```python
from build123d import *

# Parameters (mm, degrees)
EXTRUDE_1_DEPTH          = 11.5
CUT_EXTRUDE_1_DEPTH      = 220.099292559
CUT_EXTRUDE_1_DEPTH_BACK = 220.099292559
CUT_EXTRUDE_3_DEPTH      = 10


with BuildPart() as part:
    # 草图2 → 凸台-拉伸1 (new body)
    with BuildSketch(Plane(origin=(0, 0, 0), x_dir=(1, 0, 0), z_dir=(0, 1, 0))):
        with BuildLine():
            Line((-167, 104), (167, 104))
            ThreePointArc((167, 104), (185.03122292, 96.53122292), (192.5, 78.5))
            Line((192.5, 78.5), (192.5, -78.5))
            ThreePointArc((192.5, -78.5), (185.03122292, -96.53122292), (167, -104))
            Line((167, -104), (-167, -104))
            ThreePointArc((-167, -104), (-185.03122292, -96.53122292), (-192.5, -78.5))
            Line((-192.5, -78.5), (-192.5, 78.5))
            ThreePointArc((-192.5, 78.5), (-185.03122292, 96.53122292), (-167, 104))
        make_face()
    extrude(amount=EXTRUDE_1_DEPTH)

    # 草图3 → 切除-拉伸1 (cut, two sides: drawn at the far end of the back side and taken through both)
    with BuildSketch(Plane(origin=(0, 11.5, 0), x_dir=(1, 0, 0), z_dir=(0, 1, 0)).offset(-CUT_EXTRUDE_1_DEPTH_BACK)):
        with BuildLine():
            Line((-167, 96.5), (167, 96.5))
            ThreePointArc((167, 96.5), (179.727922061, 91.227922061), (185, 78.5))
            Line((185, 78.5), (185, -78.5))
            ThreePointArc((185, -78.5), (179.727922061, -91.227922061), (167, -96.5))
            Line((167, -96.5), (-167, -96.5))
            ThreePointArc((-167, -96.5), (-179.727922061, -91.227922061), (-185, -78.5))
            Line((-185, -78.5), (-185, 78.5))
            ThreePointArc((-185, 78.5), (-179.727922061, 91.227922061), (-167, 96.5))
        make_face()
    extrude(amount=CUT_EXTRUDE_1_DEPTH + CUT_EXTRUDE_1_DEPTH_BACK, mode=Mode.SUBTRACT)

    # 草图6 → 切除-拉伸3 (cut)
    with BuildSketch(Plane(origin=(0, 11.5, 0), x_dir=(1, 0, 0), z_dir=(0, 1, 0))):
        with BuildLine():
            Line((-167, 101.5), (167, 101.5))
            ThreePointArc((167, 101.5), (183.263455967, 94.763455967), (190, 78.5))
            Line((190, 78.5), (190, -78.5))
            ThreePointArc((190, -78.5), (183.263455967, -94.763455967), (167, -101.5))
            Line((167, -101.5), (-167, -101.5))
            ThreePointArc((-167, -101.5), (-183.263455967, -94.763455967), (-190, -78.5))
            Line((-190, -78.5), (-190, 78.5))
            ThreePointArc((-190, 78.5), (-183.263455967, 94.763455967), (-167, 101.5))
        make_face()
        with BuildLine():
            Line((-167, 99), (167, 99))
            ThreePointArc((167, 99), (181.495689014, 92.995689014), (187.5, 78.5))
            Line((187.5, 78.5), (187.5, -78.5))
            ThreePointArc((187.5, -78.5), (181.495689014, -92.995689014), (167, -99))
            Line((167, -99), (-167, -99))
            ThreePointArc((-167, -99), (-181.495689014, -92.995689014), (-187.5, -78.5))
            Line((-187.5, -78.5), (-187.5, 78.5))
            ThreePointArc((-187.5, 78.5), (-181.495689014, 92.995689014), (-167, 99))
        make_face(mode=Mode.SUBTRACT)
    extrude(amount=-CUT_EXTRUDE_3_DEPTH, mode=Mode.SUBTRACT)


solid = part.part
```
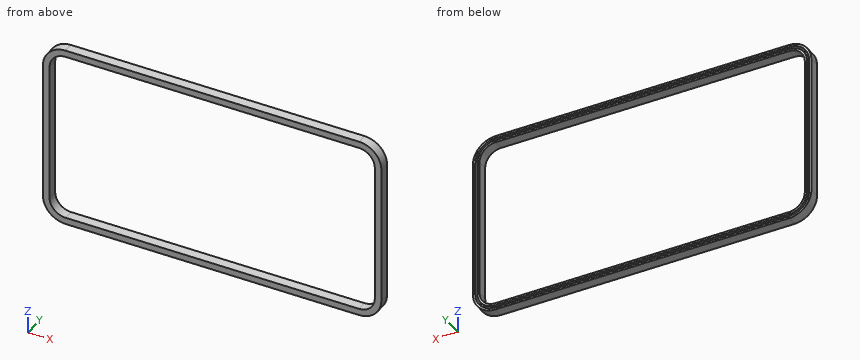
Work out the finished part from the listing and answer in its coordinate system (mm). Give positions to 0.01 mm unless a question says otherwise; leave off trailing zeros. Order: outer loops, then holes, each group sorted by start corner. A loop starts at its lowest first (then second) coordinate and runs counter-clockwise, first axis right, second up.
1. Section A-A, the plane y = 6.25 is taken. Give the number of separate pieces and of enclosed holes in the cut face, and give its area (3 significant figures).
Result sheet:
separate pieces: 2
enclosed holes: 2
area: 5,590 mm2
2. Straight lines are drawn through the part: L1, parallel to Z at x = -66, y = 7.75; L2, parallel to X at y = 8.75, z = -27; L3, parallel to Z at x = 168.5, y = 3.5. For each, find the intervals that lie inside material, in ascending order.
Result sheet:
L1: z = -104 to -101.5, -99 to -96.5, 96.5 to 99, 101.5 to 104
L2: x = -192.5 to -190, -187.5 to -185, 185 to 187.5, 190 to 192.5
L3: z = -103.96 to -101.45, -98.95 to -96.44, 96.44 to 98.95, 101.45 to 103.96
3. Section B-B, the plane z = -39 is taken. Determine the outline of the cut face in (x, y).
Result sheet:
outline: (-192.5, 0) - (-185, 0) - (-185, 11.5) - (-187.5, 11.5) - (-187.5, 1.5) - (-190, 1.5) - (-190, 11.5) - (-192.5, 11.5) - close; (185, 0) - (192.5, 0) - (192.5, 11.5) - (190, 11.5) - (190, 1.5) - (187.5, 1.5) - (187.5, 11.5) - (185, 11.5) - close
4. Section C-C, the plane x = 155 is taken. Determine the outline of the cut face in (y, z), and give its area (4 significant figures).
Result sheet:
outline: (0, -104) - (11.5, -104) - (11.5, -101.5) - (1.5, -101.5) - (1.5, -99) - (11.5, -99) - (11.5, -96.5) - (0, -96.5) - close; (0, 96.5) - (11.5, 96.5) - (11.5, 99) - (1.5, 99) - (1.5, 101.5) - (11.5, 101.5) - (11.5, 104) - (0, 104) - close
area: 122.5 mm2
